from build123d import *

# Parameters (mm, degrees)
F0_W     = 120
F0_H     = 120
F1_DEPTH = 30
F2_R     = 38.7612750812
F3_DEPTH = 25.4
F4_R     = 32.4112735689
F5_DEPTH = 55.401
F6_R     = 12.7
F7_R     = 5.08
F8_T     = -2.54


with BuildPart() as f1:
    # F0 (on Front) → F1 (new body)
    with BuildSketch(Plane.XZ):
        Rectangle(F0_W, F0_H)
    extrude(amount=F1_DEPTH)

    # F2 (on face) → F3 (join)
    with BuildSketch(Plane.XZ.offset(30)):
        Circle(F2_R)
    extrude(amount=F3_DEPTH)

    # F4 (on face) → F5 (cut, through all)
    with BuildSketch(Plane.XZ.offset(55.4)):
        Circle(F4_R)
    extrude(amount=-F5_DEPTH, mode=Mode.SUBTRACT)

    # F6
    f6_edges = [f1.edges().sort_by_distance(p)[0] for p in [
        (-60, -15, -60),
        (-60, -15, 60),
        (60, -15, 60),
        (60, -15, -60),
    ]]
    fillet(f6_edges, radius=F6_R)

    # F7
    f7_edges = [f1.edges().sort_by_distance(p)[0] for p in [
        (0, -30, -60),
        (-56.280256, -30, -56.280256),
        (56.280256, -30, -56.280256),
        (-60, -30, 0),
        (60, -30, 0),
        (-56.280256, -30, 56.280256),
        (56.280256, -30, 56.280256),
        (0, -30, 60),
        (-38.761275, -30, 0),
    ]]
    fillet(f7_edges, radius=F7_R)

    # F8
    f8_openings = [f1.faces().sort_by_distance(p)[0] for p in [
        (0, 0, -58.302944),
    ]]
    offset(amount=F8_T, openings=f8_openings)


solid = f1.part
Source: CAD feature listing. Evaluate the final solid. Frame: model axes, mm. A direction names the side the tool comes from. Give positions to 0.01 mm unless a question says otherwise; leave off trailing zeros. Order: outer loops, then holes, each group sorted by start corner. A loop starts at its lowest first (then second) coordinate and runs counter-clockwise, first axis right, second up. Notation, with made-up numbers: (-32.75, 65.25) -> (-5.75, 65.25) arc R29 ccw to (-5.75, 100.25) -> close; hole circle Ø7 at (-22.5, -27). An arc over 180 degrees is marked (long way). Use a Markdown table: item, result.
1) Contact query for flat-ended pins moving along their axis: P1, Ø2, axis at y = -28.5, z = 38.5, coming from the +X side; P2, Ø8, axis at y = -38, z = 21.5, coming from the +X side; P3, Ø3, axis at x = 16, z = -37.5, coming from the -Y side. Output: stop coordinate, or through.
Answer list:
| item | result |
|---|---|
| P1 | x = 59.3 |
| P2 | x = 34.59 |
| P3 | y = -32.86 |
2) Section query D-D, the plane y = -49. Return the cut outline in (x, z).
Answer list:
| item | result |
|---|---|
| outline | circle Ø77.52 at (0, 0); circle Ø69.9 at (0, 0); hole circle Ø72.44 at (0, 0); hole circle Ø64.82 at (0, 0) |
3) Section query B-B, the plane y = -22.5. Return the cut outline in (x, z), then the cut area to 3 significant figures.
Answer list:
| item | result |
|---|---|
| outline | (-60, -47.3) arc R12.7 ccw to (-47.3, -60) -> (47.3, -60) arc R12.7 ccw to (60, -47.3) -> (60, 47.3) arc R12.7 ccw to (47.3, 60) -> (-47.3, 60) arc R12.7 ccw to (-60, 47.3) -> close; circle Ø69.9 at (0, 0); hole (-57.46, -47.3) arc R10.16 ccw to (-47.3, -57.46) -> (47.3, -57.46) arc R10.16 ccw to (57.46, -47.3) -> (57.46, 47.3) arc R10.16 ccw to (47.3, 57.46) -> (-47.3, 57.46) arc R10.16 ccw to (-57.46, 47.3) -> close; hole circle Ø64.82 at (0, 0) |
| area | 1,680 mm² |
4) Mould query, pull axis X, two halves, no side actions, for faces 4 (the cylindrical face through (-58.472, -28.551, -0.662)), 5 (the cylindrical face through (54.405, -12.634, -54.563)), 6 (the flat face through (31, 0, -10)). Classes: +X half, -X half, draft (parallel to the pull), parting line (faces both ways), or undercut.
Answer list:
| item | result |
|---|---|
| face 4 | -X half |
| face 5 | undercut |
| face 6 | draft |
5) Ray query, line 1 along Z through (x, y) = (0, -44.25); line 2 along X through (y, z) = (-15.5, 17.5); line 3 along Z through (x, y) = (-13, -16). Return the intervals inside material, ascending. Write a range as [from, to].
Answer list:
| item | result |
|---|---|
| line 1 | [-38.76, -36.22], [-34.95, -32.41], [32.41, 34.95], [36.22, 38.76] |
| line 2 | [-60, -57.46], [-30.25, -27.28], [27.28, 30.25], [57.46, 60] |
| line 3 | [-60, -57.46], [-32.44, -29.69], [29.69, 32.44], [57.46, 60] |
6) Reachability of faces 1 (the flat face through (-25, -30, 37)), 2 (the flat face through (-25, -27.46, 37)), 3 (the cylindrical face through (58.472, -28.551, 0.662)) from +Z, -Z, +X, -X, +Y, -Y: full face, straight path, thin tool, end or side. Return the list, or none.
Answer list:
| item | result |
|---|---|
| face 1 | -Y |
| face 2 | +Y |
| face 3 | +Z, -Z, +X, -Y |
